from build123d import *

# Parameters (mm, degrees)
SKETCH1_W           = 40
SKETCH1_H           = 40
SKETCH1_W_2         = 29
SKETCH1_H_2         = 29
BOSS_EXTRUDE1_DEPTH = 25
SKETCH2_W           = 40
SKETCH2_H           = 40
SKETCH2_W_2         = 32
SKETCH2_H_2         = 32
BOSS_EXTRUDE2_DEPTH = 10
SKETCH4_W           = 80
SKETCH4_H           = 40
SKETCH4_W_2         = 29
SKETCH4_H_2         = 29
BOSS_EXTRUDE3_DEPTH = 5
FILLET6_R           = 5


with BuildPart() as part:
    # Sketch1 → Boss-Extrude1 (new body)
    with BuildSketch(Plane(origin=(0, 0, 0), x_dir=(1, 0, 0), z_dir=(0, 1, 0))):
        with Locations((20, 20)):
            Rectangle(SKETCH1_W, SKETCH1_H)
        with Locations((20, 20)):
            Rectangle(SKETCH1_W_2, SKETCH1_H_2, mode=Mode.SUBTRACT)
    extrude(amount=BOSS_EXTRUDE1_DEPTH)

    # Sketch2 → Boss-Extrude2 (add)
    with BuildSketch(Plane(origin=(0, 25, 0), x_dir=(1, 0, 0), z_dir=(0, 1, 0))):
        with Locations((20, 20)):
            Rectangle(SKETCH2_W, SKETCH2_H)
        with Locations((20, 20)):
            Rectangle(SKETCH2_W_2, SKETCH2_H_2, mode=Mode.SUBTRACT)
    extrude(amount=BOSS_EXTRUDE2_DEPTH)

    # Sketch4 → Boss-Extrude3 (add)
    with BuildSketch(Plane.XZ):
        with Locations((20, -20)):
            Rectangle(SKETCH4_W, SKETCH4_H)
        with Locations((20, -20)):
            Rectangle(SKETCH4_W_2, SKETCH4_H_2, mode=Mode.SUBTRACT)
    extrude(amount=BOSS_EXTRUDE3_DEPTH)

    # Fillet6
    fillet6_edges = [part.edges().sort_by_distance(p)[0] for p in [
        (5.5, 10, -5.5),
        (34.5, 10, -5.5),
        (34.5, 10, -34.5),
        (5.5, 10, -34.5),
        (0, 17.5, -40),
        (40, 17.5, -40),
        (40, 17.5, 0),
        (0, 17.5, 0),
    ]]
    fillet(fillet6_edges, radius=FILLET6_R)


solid = part.part
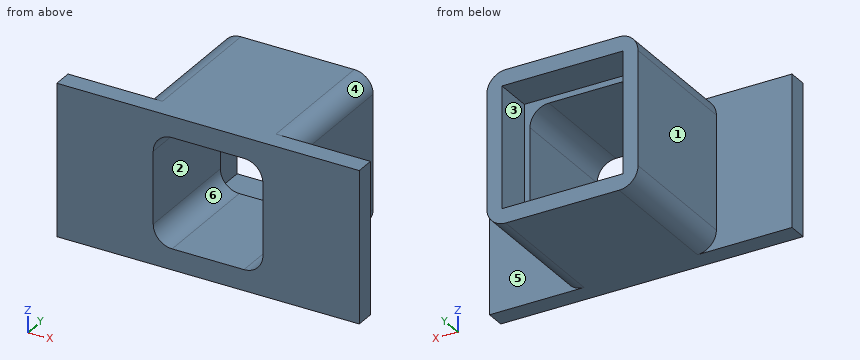
Could you check a few things on this model? Use its own coordinates, in mm. Face numbers are marked on the shaded views. A direction names the side the tool comes from. Give positions to 0.01 mm unless a question says otherwise; leave off trailing zeros. Order: outer loops, then holes, each group sorted by start corner. A loop starts at its lowest first (then second) coordinate and runs counter-clockwise, first axis right, second up. Notation, with made-up numbers: (73.25, 71) -> (116.25, 71) arc R32 cw to (116.25, 106) -> close; hole circle Ø8 at (60, 16.5). An arc over 180 degrees is marked (long way). Return JSON: item names as keys, results as strings.
1. Imagine slicing it at C-C on x = 19. List the corners of the cut face in (y, z) for me.
Answer list:
{"outline": "(-5, -40) -> (35, -40) -> (35, -36) -> (25, -36) -> (25, -34.5) -> (-5, -34.5) -> close; (-5, -5.5) -> (25, -5.5) -> (25, -4) -> (35, -4) -> (35, 0) -> (-5, 0) -> close"}
2. On a 3-axis mill with a long thin cutter (end or side, diameter ignored), from which of +Z, -Z, +X, -X, +Y, -Y can I reach the whole of each face in a straight line? I mean the marked faces 1, 2 and 3. Say none if no direction works.
Answer list:
{"face 1": "+Z, -Z, -X, +Y", "face 2": "+Y, -Y", "face 3": "+Y"}
3. Imagine slicing it at B-B on y = 26. List the corners of the cut face in (x, z) for me, then the cut area to 3 significant figures.
Answer list:
{"outline": "(0, -35) arc R5 ccw to (5, -40) -> (35, -40) arc R5 ccw to (40, -35) -> (40, -5) arc R5 ccw to (35, 0) -> (5, 0) arc R5 ccw to (0, -5) -> close; hole (4, -36) -> (36, -36) -> (36, -4) -> (4, -4) -> close", "area": "555 mm2"}
4. I need wall thicknesses on line 1 (X direction, y = 30.5, z = -14.5); line 2 (Z direction, x = 27, y = 29); line 3 (Z direction, x = 22, y = 8.5). Which ranges of each line are inside material? Lowest first, please. Write a range as from..to.
Answer list:
{"line 1": "x = 0..4, 36..40", "line 2": "z = -40..-36, -4..0", "line 3": "z = -40..-34.5, -5.5..0"}
5. For pin 1 Ø1 at (y, z) = (15.5, -19.5) entering from -X; pin 2 Ø12.5 at (x, z) = (-10, -29.5) entering from +Y; pin 3 Ø3 at (y, z) = (29, -13) entering from +X, each with a flat end and sliding along its axis, tell me the tip position at first contact or that it passes through.
Answer list:
{"pin 1": "stops at x = 0", "pin 2": "stops at y = 0", "pin 3": "stops at x = 40"}
6. Thinking about a two-plate mould opening in Z: for the marked faces 4, 5 and 6, which applies, pulls with the +Z half, pulls with the -Z half, needs draft (parallel to the pull), parting line crosses it, or undercut?
Answer list:
{"face 4": "pulls with the +Z half", "face 5": "needs draft", "face 6": "undercut"}
7. Imagine slicing it at A-A on z = -17. List the corners of the cut face in (x, y) for me, then the cut area to 3 significant figures.
Answer list:
{"outline": "(-20, -5) -> (5.5, -5) -> (5.5, 25) -> (4, 25) -> (4, 35) -> (0, 35) -> (0, 0) -> (-20, 0) -> close; (34.5, -5) -> (60, -5) -> (60, 0) -> (40, 0) -> (40, 35) -> (36, 35) -> (36, 25) -> (34.5, 25) -> close", "area": "610 mm2"}
8. Imagine slicing it at D-D on y = -1.5. List the corners of the cut face in (x, z) for me, then the cut area to 3 significant figures.
Answer list:
{"outline": "(-20, -40) -> (60, -40) -> (60, 0) -> (-20, 0) -> close; hole (5.5, -29.5) arc R5 ccw to (10.5, -34.5) -> (29.5, -34.5) arc R5 ccw to (34.5, -29.5) -> (34.5, -10.5) arc R5 ccw to (29.5, -5.5) -> (10.5, -5.5) arc R5 ccw to (5.5, -10.5) -> close", "area": "2,380 mm2"}
